Source: CAD feature listing. Evaluate the final solid. Frame: model axes, mm. A direction names the side the tool comes from. Round coordinates to 2 decimals unless told otherwise and drop trailing zeros. Loops run counter-clockwise (first coordinate to the right, second up) from the corner with the lowest first, then second, coordinate; pieces in that order, holes last. Notation, with made-up numbers: M 21,86 L 43,86 A20 cw 43,94 Z; hole C 12,73.5 d9. An arc over 180 degrees is marked long. Answer as CSV lines item,"result". Start each with the question number.
```python
from build123d import *

# Parameters (mm, degrees)
SKETCH_1_W      = 30
SKETCH_1_H      = 34
EXTRUDE_1_DEPTH = 25
SKETCH_2_R      = 11.5
EXTRUDE_2_DEPTH = 17


with BuildPart() as part:
    # 草图1 → 凸台-拉伸1 (new body)
    with BuildSketch(Plane.XY):
        Rectangle(SKETCH_1_W, SKETCH_1_H)
    extrude(amount=EXTRUDE_1_DEPTH)

    # 草图2 → 凸台-拉伸2 (add)
    with BuildSketch(Plane.XY.offset(25)):
        Circle(SKETCH_2_R)
    extrude(amount=EXTRUDE_2_DEPTH)

    # 草图3 → 旋转1 (revolve)
    with BuildSketch(Plane(origin=(0, 0, 0), x_dir=(1, 0, 0), z_dir=(0, 1, 0))):
        with BuildLine():
            Line((0, -42), (15, -42))
            Line((15, -42), (15, -44))
            ThreePointArc((15, -44), (8.618709266, -50.222281386), (0, -52.492855685))
            Line((0, -52.492855685), (0, -42))
        make_face()
    revolve(axis=Axis((0, 0, 42), (0, 0, 1)))


solid = part.part
```
1) Section A-A, the plane y = 0. Return loops of the section in (x, z).
2) Section C-C, the plane x = 0. Return loops of the section in (y, z).
3) Access query for faces 4 (the flat face through (15, 0, 12)), 5 (the flat face through (-8, -9, 42)), 6 (the cylindrical face through (-14.985, 0.66, 43.014)). Directions: +Z, -Z, +X, -X, +Y, -Y. A direction counts if a zero-diameter tool reaches every point of the face in a straight line with its end or side. Return the directions, or none.
4) Section D-D, the plane z = 28.5. Return loops of the section in (x, y).
5) Ray query, line 1 along Z through (x, y) = (-2.5, -13); line 2 along Z through (x, y) = (9.75, 15.5); line 3 along Z through (x, y) = (-11, -3.5). Return the intervals inside material, ascending.
6) Contact query for flat-ended pins moving along their axis: pin 1 Ø3 at (y, z) = (10, 47) entering from +X; pin 2 Ø5 at (x, z) = (2.5, 31) entering from -Y; pin 3 Ø10 at (x, z) = (6.5, 33) entering from -Y. Output: stop coordinate, or through.
7) Section B-B, the plane y = 12.5. Return loops of the section in (x, z).
8) Mould query, pull axis Z, two halves, no side actions, for faces 1 (the flat face through (0, 0, 0)), 2 (the flat face through (0, 12, 25)), 3 (the flat face through (0, 17, 12)). Classes: pulls with the +Z half, pulls with the -Z half, needs draft (parallel to the pull), parting line crosses it, or undercut.
Findings below:
1,outline,"M -15,0 L 15,0 L 15,25 L 11.5,25 L 11.5,42 L 15,42 L 15,44 A17.49 ccw -15,44 L -15,42 L -11.5,42 L -11.5,25 L -15,25 Z"
2,outline,"M -17,0 L 17,0 L 17,25 L 11.5,25 L 11.5,42 L 15,42 L 15,44 A17.49 ccw -15,44 L -15,42 L -11.5,42 L -11.5,25 L -17,25 Z"
3,face 4,"+Z, -Z, +X, +Y, -Y"
3,face 5,"none"
3,face 6,"+Z"
4,outline,"C 0,0 d23"
5,line 1,"0 to 25, 42 to 46.43"
5,line 2,"0 to 25"
5,line 3,"0 to 25, 42 to 48.14"
6,pin 1,"x = 10.33"
6,pin 2,"y = -11.5"
6,pin 3,"y = -11.4"
7,outline,"M -15,0 L 15,0 L 15,25 L -15,25 Z; M -8.29,42 L 8.29,42 L 8.29,44 A12.24 ccw -8.29,44 Z"
8,face 1,"pulls with the -Z half"
8,face 2,"undercut"
8,face 3,"needs draft"
